Study the drawing (mm; zero at the part's minimum x, y, z) and answer. A direction names the side the tool comes from. Round coordinates to 2 decimals unless told otherwise and drop trailing zeros. Write each loop counter-clockwise with the first axis right and the second up, starting at its lowest first coordinate (ties: lowest second). Pieces come first, ordered by that corner, then holes.
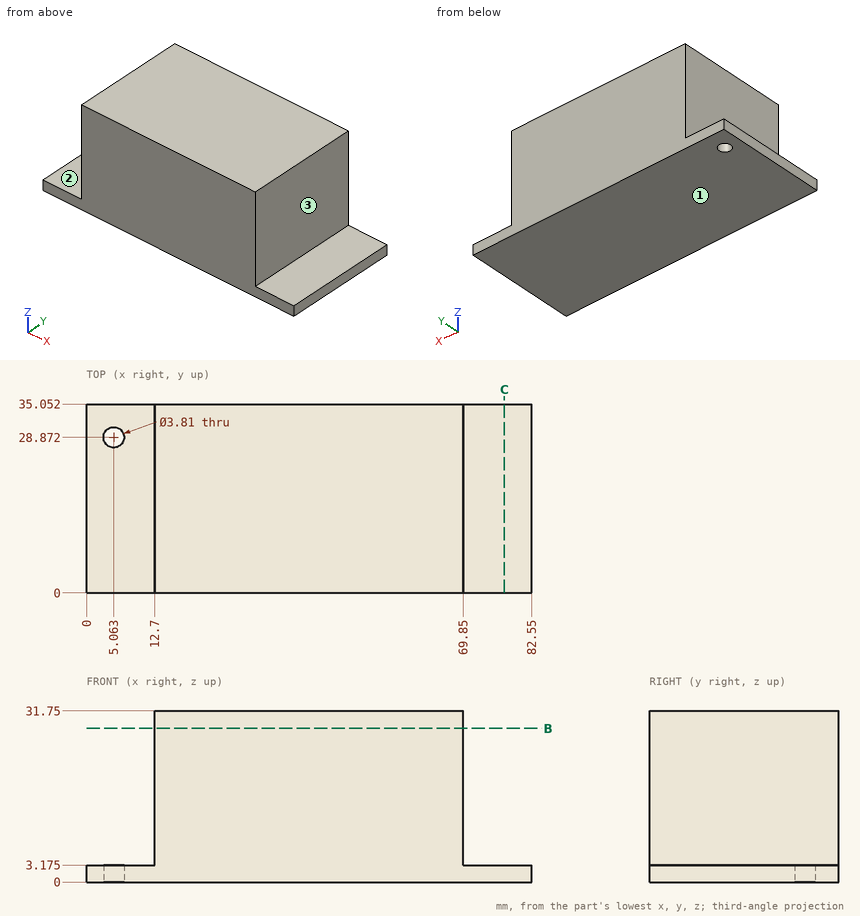
Q1. Find section C-C (x = 77.5). Determine the outline of the cut face in (y, z) (1 decimal).
Q2. Find section B-B (z = 28.5). Determine the outline of the cut face in (x, y).
Q3. A tool of negligible diameter and unlimited length cuts with its end or side. For the marked faces 1, 2 and 3, from which of +Z, -Z, +X, -X, +Y, -Y can it reach the whole face along a straight path? Write none if from no direction.
Q4. Find the intervals of material crossed by L1, parallel to X at y = 25.5, z = 4; L2, parallel to Z at x = 77, y = 32.5 (1 decimal), in increasing order.
Q5. Given pin 1 (10 mm diameter, centred on x = 7, y = 26, fed in from +Z) (3 decimals); pin 2 (1.5 mm diameter, centred on y = 22.5, z = 24.5, fed in from +X); pin 3 (2 mm diameter, centred on y = 8.5, z = 14, fed in from -X), each flat-ended and moving along its own axis, determine where each tip first touches the part or whether it passes through.
Report:
1. outline: (0, 0) - (35.1, 0) - (35.1, 3.2) - (0, 3.2) - close
2. outline: (12.7, 0) - (69.85, 0) - (69.85, 35.05) - (12.7, 35.05) - close
3. face 1: -Z, +X, -X, +Y, -Y
3. face 2: +Z, -X, +Y, -Y
3. face 3: +Z, +X, +Y, -Y
4. L1: x = 12.7 to 69.85
4. L2: z = 0 to 3.2
5. pin 1: stops at z = 3.175
5. pin 2: stops at x = 69.85
5. pin 3: stops at x = 12.7
